```python
from build123d import *

# Parameters (mm, degrees)
F2_R    = 0.508
F3_SIZE = 0.508


with BuildPart() as f1:
    # F0 (on Front) → F1 (revolve)
    with BuildSketch(Plane.XZ):
        Polygon((-12.7, 0), (0, 0), (0, 6.35), (-3.416564, 4.876191), (-4.833689, 3.118957), (-7.157773, 3.118957), (-8.574897, 4.876191), (-10.388815, 4.876191), (-11.125719, 6.35), (-12.7, 6.35), align=None)
    revolve(axis=Axis((-6.35, 0, 0), (-1, 0, 0)))

    # F2
    f2_edges = [f1.edges().sort_by_distance(p)[0] for p in [
        (0, 0, -6.35),
        (-3.416564, 0, -4.876191),
        (-8.574897, 0, -4.876191),
        (-11.125719, 0, -6.35),
    ]]
    fillet(f2_edges, radius=F2_R)

    # F3
    f3_edges = [f1.edges().sort_by_distance(p)[0] for p in [
        (-12.7, 0, -6.35),
    ]]
    chamfer(f3_edges, length=F3_SIZE)


solid = f1.part
```
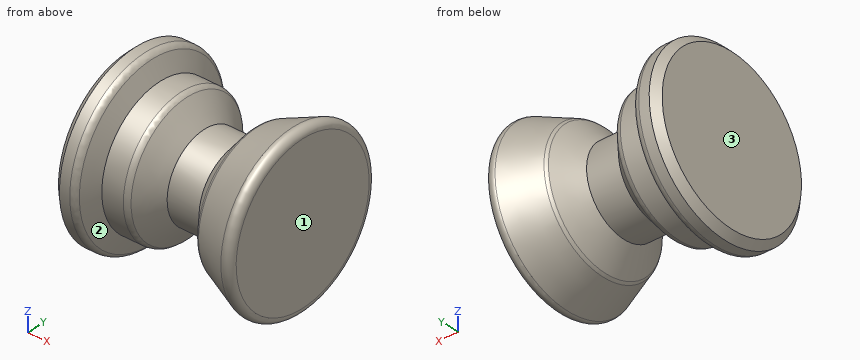
Work out the finished part from the listing and answer in its coordinate system (mm). Face numbers are marked on the shaded views. Coordinates: 2 decimals unless noted, no trailing zeros. Loops run counter-clockwise (first coordinate to the right, second up) from the corner with the lowest first, then second, coordinate; pieces in that order, holes last. Notation, with made-up numbers: (16.5, 10) - (59.5, 10) arc R23 ccw to (59.5, 24) - close; hole circle Ø3 at (-38, -10). An arc over 180 degrees is marked (long way). Use a Markdown table: item, result.
Item 1: Given pin 1 Ø5 at (x, z) = (-11.5, -5) entering from +Y; pin 2 Ø5 at (x, y) = (-3.5, -2.5) entering from +Z; pin 3 Ø1.5 at (x, y) = (-10.5, 0.5) entering from -Z, each flat-ended and moving along its own axis, determine where each tip first touches the part or whether it passes through.
Evaluation:
| item | result |
|---|---|
| pin 1 | stops at y = 5.84 |
| pin 2 | stops at z = 5.64 |
| pin 3 | stops at z = -6.3 |
Item 2: The mould has two halves that part along X. Classify the marked faces 1, 2 and 3: +X half, -X half, draft (parallel to the pull), parting line (faces both ways), or undercut.
Evaluation:
| item | result |
|---|---|
| face 1 | +X half |
| face 2 | undercut |
| face 3 | -X half |
Item 3: Find section A-A, the plane x = -5.5. Determine the outline of the cut face in (y, z), and give its area (3 significant figures).
Evaluation:
| item | result |
|---|---|
| outline | circle Ø6.24 at (0, 0) |
| area | 30.6 mm2 |
Item 4: Consider probe 1 along X at (y, z) = (2.5, -5.25); probe 2 along X at (y, z) = (3.75, -2.75); probe 3 along Y at (x, z) = (-3, -4). Determine where each line is inside the solid, lowest interval first. Write a range as from..to.
Evaluation:
| item | result |
|---|---|
| probe 1 | x = -12.7..-10.86, -1.24..-0.06 |
| probe 2 | x = -12.7..-8.39, -3.6..0 |
| probe 3 | y = -3.09..3.09 |
Item 5: Find section B-B, the plane x = -3.75. Determine the outline of the cut face in (y, z).
Evaluation:
| item | result |
|---|---|
| outline | circle Ø8.93 at (0, 0) |
